from build123d import *

# Parameters (mm, degrees)
F1_DEPTH = 50.8


with BuildPart() as f1:
    # F0 (on Front) → F1 (new body)
    with BuildSketch(Plane.XZ):
        Polygon((0, 47.668528), (-25.4, 3.674437), (-6.35, 3.674437), (25.4, 3.674437), align=None)
        with BuildLine():
            Line((-6.35, 3.674437), (-25.4, 3.674437))
            Line((-25.4, 3.674437), (-25.4, -28.075563))
            Line((-25.4, -28.075563), (-13.173735, -28.075563))
            ThreePointArc((-13.173735, -28.075563), (-11.17511, -23.250453), (-6.35, -21.251827))
            Line((-6.35, -21.251827), (-6.35, 3.674437))
        make_face()
        with BuildLine():
            Line((25.4, 3.674437), (-6.35, 3.674437))
            Line((-6.35, 3.674437), (-6.35, -21.251827))
            ThreePointArc((-6.35, -21.251827), (-1.52489, -23.250453), (0.473735, -28.075563))
            Line((0.473735, -28.075563), (25.4, -28.075563))
            Line((25.4, -28.075563), (25.4, 3.674437))
        make_face()
        with BuildLine():
            Line((-13.173735, -28.075563), (-25.4, -28.075563))
            Line((-25.4, -28.075563), (-25.4, -47.125563))
            Line((-25.4, -47.125563), (-6.35, -47.125563))
            Line((-6.35, -47.125563), (-6.35, -34.899298))
            ThreePointArc((-6.35, -34.899298), (-11.17511, -32.900672), (-13.173735, -28.075563))
        make_face()
        with BuildLine():
            Line((25.4, -47.125563), (25.4, -28.075563))
            Line((25.4, -28.075563), (0.473735, -28.075563))
            ThreePointArc((0.473735, -28.075563), (-1.52489, -32.900672), (-6.35, -34.899298))
            Line((-6.35, -34.899298), (-6.35, -47.125563))
            Line((-6.35, -47.125563), (25.4, -47.125563))
        make_face()
    extrude(amount=F1_DEPTH)


solid = f1.part
Geometry check sheet. Reference: the model listing, model coordinates, mm. Give positions to 0.01 mm unless a question says otherwise; leave off trailing zeros. Order: outer loops, then holes, each group sorted by start corner. A loop starts at its lowest first (then second) coordinate and runs counter-clockwise, first axis right, second up.
1. Scan lines: line 1 (Z direction, x = -12.5, y = -5); line 2 (Z direction, x = -4, y = -13.5); line 3 (X direction, y = -26.5, z = -30.5). Record each from-to range of solid material in increasing order.
Completed:
line 1: z = -47.13 to -31.03, -25.12 to 26.02
line 2: z = -47.13 to -34.48, -21.67 to 40.74
line 3: x = -25.4 to -12.73, 0.03 to 25.4
2. Sectioned sample at C-C (y = -41.5). Record the boundary of the cut face in (x, z), then the cut area to 3 significant figures.
Completed:
outline: (-25.4, -47.13) - (25.4, -47.13) - (25.4, 3.67) - (0, 47.67) - (-25.4, 3.67) - close; hole (-13.17, -28.08) arc R6.82 ccw to (-6.35, -34.9) arc R6.82 ccw to (0.47, -28.08) arc R6.82 ccw to (-6.35, -21.25) arc R6.82 ccw to start
area: 3,550 mm2
3. Sectioned sample at D-D (x = 16). Record the boundary of the cut face in (y, z), then the cut area to 3 significant figures.
Completed:
outline: (-50.8, -47.13) - (0, -47.13) - (0, 19.96) - (-50.8, 19.96) - close
area: 3,410 mm2
4. Sectioned sample at B-B (z = -23). Record the boundary of the cut face in (x, y), then the cut area to 3 significant figures.
Completed:
outline: (-25.4, -50.8) - (-10.91, -50.8) - (-10.91, 0) - (-25.4, 0) - close; (-1.79, -50.8) - (25.4, -50.8) - (25.4, 0) - (-1.79, 0) - close
area: 2,120 mm2
5. Depth check by flat-ended pin: pin 1 (12 mm diameter, centred on y = -19, z = 31, fed in from -X); pin 2 (8 mm diameter, centred on x = 2.5, y = -15, fed in from +Z); pin 3 (10 mm diameter, centred on x = -15.5, y = -8.5, fed in from +Z). Enter the tip coordinate at first touch or a pass-through.
Completed:
pin 1: stops at x = -13.09
pin 2: stops at z = 47.67
pin 3: stops at z = 29.48
6. Sectioned sample at A-A (x = -1.5). Record the boundary of the cut face in (y, z).
Completed:
outline: (-50.8, -47.13) - (0, -47.13) - (0, -32.88) - (-50.8, -32.88) - close; (-50.8, -23.28) - (0, -23.28) - (0, 45.07) - (-50.8, 45.07) - close
